For this review, take the finished solid that the model builds, in its own axes (mm). A direction names the side the tool comes from. Give positions to 0.01 mm unless a question says otherwise; leave off trailing zeros. Order: outer loops, then holes, each group sorted by start corner. A loop starts at its lowest first (then second) coordinate and runs counter-clockwise, first axis right, second up. Notation, with made-up numbers: M -4,62 L 22,62 A17 cw 22,95 Z; hole C 3,-11.75 d8. An arc over 180 degrees is marked long. Use CSV: the item, a comma, the result in double quotes. Start each with the question number.
(1) Wall thickness on L1, parallel to Y at x = 67.5, z = -1; L2, parallel to Y at x = 67, z = -1.05; L3, parallel to X at y = -41, z = 0.6: over which ranges is each line inside the solid? List them lowest first. Write a range as from..to.
(2) Tool access review of faces 5 (the face through (61.27, -27.46, 0.04)), 6 (the face through (57.906, 44.229, 0.042)), 7 (the face through (60, -50, 0)): name each direction out of +Z, -Z, +X, -X, +Y, -Y from which nothing blocks a thin tool from reaching the whole face with its end or side.
(3) Consider section A-A (y = -55). Write out the cut boundary in (x, z).
(4) Draft analysis for pull direction X (two halves, no side actions). For faces 1 (the face through (60, 61, 0)), 2 (the face through (68.651, 54.957, -0.042)), 3 (the face through (68.651, -50.043, -0.042)), 4 (the face through (68, -70, 0)), state which applies: pulls with the +X half, pulls with the -X half, needs draft (parallel to the pull), parting line crosses it, or undercut.
(5) Consider section C-C (x = 64.5). Write out the cut boundary in (y, z), and give its area (3 significant figures).
(6) Clearance check with flat-ended pins moving along their axes: P1, Ø9, axis at x = 68, y = -55, coming from the -Z side; P2, Ø3, axis at y = 62, z = 1, coming from the -X side. State where each tip first meets the part, or that it passes through.
(7) Consider section D-D (y = 47). Write out the cut boundary in (x, z), and give its area (3 significant figures).
(8) Consider section B-B (z = 0.6). Write out the cut boundary in (x, y), and give its area (3 significant figures).
```python
from build123d import *

# Parameters (mm, degrees)
BOSS_EXTRUDE1_DEPTH        = 3
F_10_0_10_DIAMETER_HOLE1_D = 10


with BuildPart() as part:
    # Sketch1 → Boss-Extrude1 (new, symmetric)
    with BuildSketch(Plane.XY):
        with BuildLine():
            Line((59.999997079, 62), (59.999997079, 57))
            ThreePointArc((59.999997079, 57), (57.847096138, 44.054070414), (51.620142438, 32.501706028))
            ThreePointArc((51.620142438, 32.501706028), (60.750395332, 5.512664234), (56.627398554, -22.679015256))
            Line((56.627398554, -22.679015256), (60, -24.011943529))
            Line((60, -24.011943529), (62.5, -25))
            Line((62.5, -25), (60, -30))
            Line((60, -30), (60, -70))
            Line((60, -70), (75.999997079, -70))
            Line((75.999997079, -70), (75.999997079, 62))
            Line((75.999997079, 62), (75.999997079, 65))
            Line((75.999997079, 65), (59.999997079, 65))
            Line((59.999997079, 65), (59.999997079, 62))
        make_face()
    extrude(amount=BOSS_EXTRUDE1_DEPTH, both=True)

    # Ø10.0 (10) Diameter Hole1 (through all)
    with Locations(Plane(origin=(67.999997079, 50, 3), x_dir=(1, 0, 0), z_dir=(0, 0, 1))):
        with Locations((0, 0), (0, -105)):
            Hole(F_10_0_10_DIAMETER_HOLE1_D / 2)


solid = part.part
```
Check result:
1,L1,"y = -70..-59.97, -50.03..45.03, 54.97..65"
1,L2,"y = -70..-59.9, -50.1..45.1, 54.9..65"
1,L3,"x = 60..76"
2,face 5,"+Z, -Z, -X"
2,face 6,"+Z, -Z, -X, +Y"
2,face 7,"+Z, -Z, -X, -Y"
3,outline,"M 60,-3 L 63,-3 L 63,3 L 60,3 Z; M 73,-3 L 76,-3 L 76,3 L 73,3 Z"
4,face 1,"pulls with the -X half"
4,face 2,"undercut"
4,face 3,"undercut"
4,face 4,"needs draft"
5,outline,"M -70,-3 L -58.57,-3 L -58.57,3 L -70,3 Z; M -51.43,-3 L 46.43,-3 L 46.43,3 L -51.43,3 Z; M 53.57,-3 L 65,-3 L 65,3 L 53.57,3 Z"
5,area,"724 mm^2"
6,P1,"passes through"
6,P2,"stops at x = 60"
7,outline,"M 58.73,-3 L 64,-3 L 64,3 L 58.73,3 Z; M 72,-3 L 76,-3 L 76,3 L 72,3 Z"
7,area,"55.6 mm^2"
8,outline,"M 51.62,32.5 A61 cw 56.63,-22.68 L 62.5,-25 L 60,-30 L 60,-70 L 76,-70 L 76,65 L 60,65 L 60,57 A40 cw Z; hole C 68,-55 d10; hole C 68,50 d10"
8,area,"2,140 mm^2"
